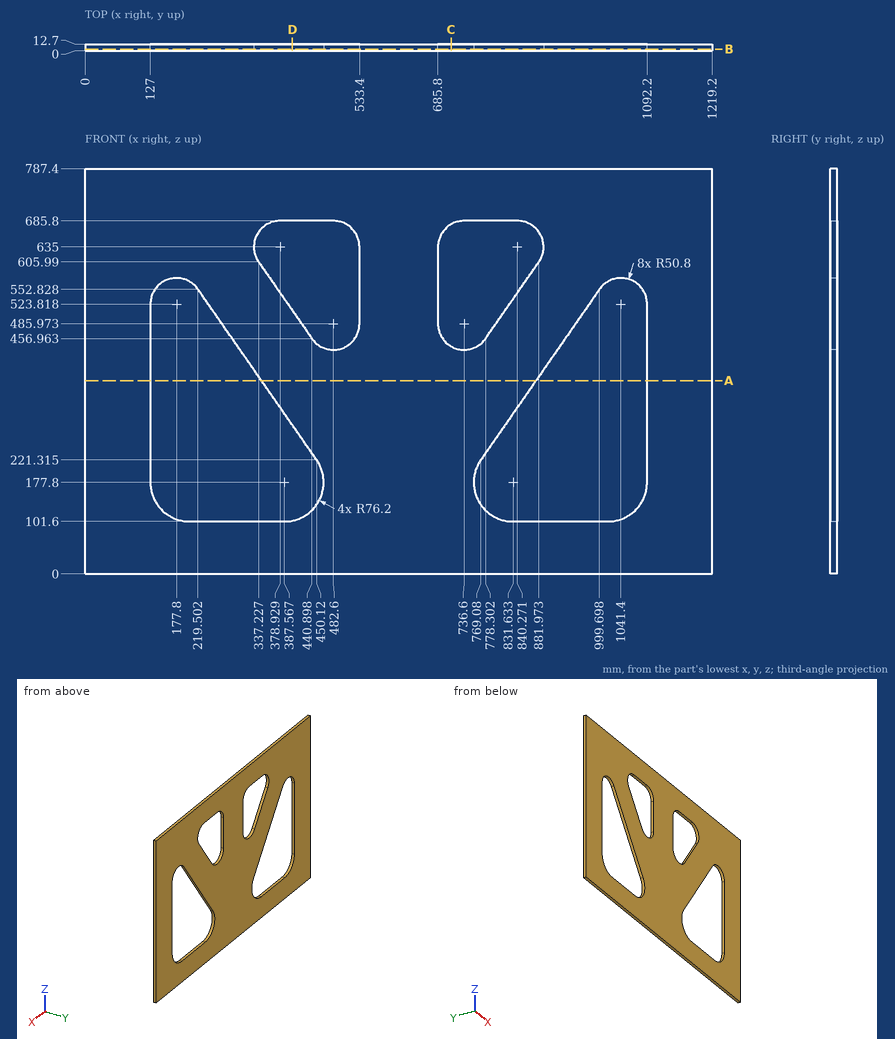
Design review of the part shown in the three views and the two pictorial views. Dimensions are in mm from the part's minimum x, y and z. Give positions to 0.01 mm unless a question says otherwise; leave off trailing zeros. Loops run counter-clockwise (first coordinate to the right, second up) from the corner with the lowest first, then second, coordinate; pieces in that order, holes last. Notation, with made-up numbers: (51.5, -22.5) - (79.5, -22.5) arc R5 cw to (79.5, -16.5) - close; hole circle Ø7 at (-25, 77). An arc over 180 degrees is marked (long way). Use CSV: the item, a comma, the result in double quotes. Start each with the question number.
1. Add section D-D (x = 403). State the section outline as (y, z) points.
2. Wall thickness on L1, parallel to Z at x = 410, y = 10 (1 decimal); L2, parallel to X at y = 4.5, z = 129 (1 decimal); L3, parallel to X at y = 5.5, z = 570 (1 decimal): over which ranges is each line inside the solid? List them lowest first.
3. Add section A-A (z = 375.5). State the section outline as (x, y) points, plus the area to 3 significant figures.
4. Add section B-B (y = 2.5). State the section outline as (x, z) points (1 decimal), plus the area to 3 significant figures.
5. Add section C-C (x = 711.5). State the section outline as (y, z) points.
Results found:
1,outline,"(0, 0) - (12.7, 0) - (12.7, 103.18) - (0, 103.18) - close; (0, 289.05) - (12.7, 289.05) - (12.7, 511.44) - (0, 511.44) - close; (0, 685.8) - (12.7, 685.8) - (12.7, 787.4) - (0, 787.4) - close"
2,L1,"z = 0 to 105, 279 to 501.4, 685.8 to 787.4"
2,L2,"x = 0 to 144.7, 446.1 to 773.1, 1074.5 to 1219.2"
2,L3,"x = 0 to 156.6, 199 to 362.3, 533.4 to 685.8, 856.9 to 1020.2, 1062.6 to 1219.2"
3,outline,"(0, 0) - (127, 0) - (127, 12.7) - (0, 12.7) - close; (342.86, 0) - (876.34, 0) - (876.34, 12.7) - (342.86, 12.7) - close; (1092.2, 0) - (1219.2, 0) - (1219.2, 12.7) - (1092.2, 12.7) - close"
3,area,"10,000 mm²"
4,outline,"(0, 0) - (1219.2, 0) - (1219.2, 787.4) - (0, 787.4) - close; hole (127, 177.8) arc R76.2 ccw to (203.2, 101.6) - (387.6, 101.6) arc R76.2 ccw to (450.1, 221.3) - (219.5, 552.8) arc R50.8 ccw to (127, 523.8) - close; hole (337.2, 606) - (440.9, 457) arc R50.8 ccw to (533.4, 486) - (533.4, 635) arc R50.8 ccw to (482.6, 685.8) - (378.9, 685.8) arc R50.8 ccw to start; hole (685.8, 486) arc R50.8 ccw to (778.3, 457) - (882, 606) arc R50.8 ccw to (840.3, 685.8) - (736.6, 685.8) arc R50.8 ccw to (685.8, 635) - close; hole (769.1, 221.3) arc R76.2 ccw to (831.6, 101.6) - (1016, 101.6) arc R76.2 ccw to (1092.2, 177.8) - (1092.2, 523.8) arc R50.8 ccw to (999.7, 552.8) - close"
4,area,"669,000 mm²"
5,outline,"(0, 0) - (12.7, 0) - (12.7, 441.81) - (0, 441.81) - close; (0, 679.17) - (12.7, 679.17) - (12.7, 787.4) - (0, 787.4) - close"
